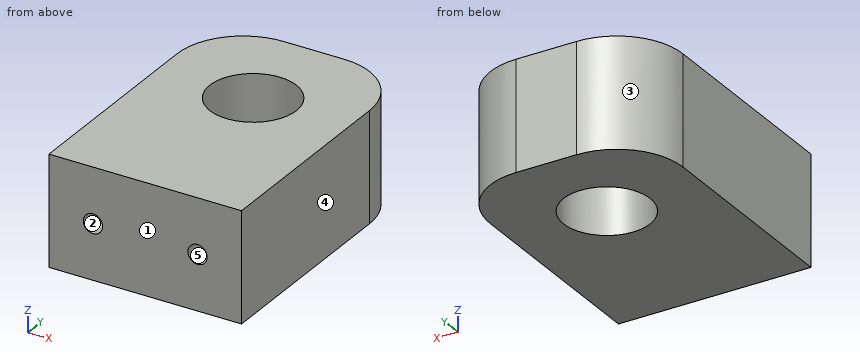
```python
from build123d import *

# Parameters (mm, degrees)
SKETCH1_W           = 35
SKETCH1_H           = 20
BOSS_EXTRUDE1_DEPTH = 50
SKETCH2_R           = 7.875
CUT_EXTRUDE1_DEPTH  = 21
SKETCH3_R           = 1.75
CUT_EXTRUDE2_DEPTH  = 10
FILLET1_R           = 12


with BuildPart() as part:
    # Sketch1 → Boss-Extrude1 (new body)
    with BuildSketch(Plane(origin=(0, 0, 0), x_dir=(1, 0, 0), z_dir=(0, 1, 0))):
        with Locations((1.164675851, -0.855170824)):
            Rectangle(SKETCH1_W, SKETCH1_H)
    extrude(amount=BOSS_EXTRUDE1_DEPTH)

    # Sketch2 → Cut-Extrude1 (cut, through all)
    with BuildSketch(Plane.XY.offset(10.855170824)):
        with Locations((1.164675851, 32)):
            Circle(SKETCH2_R)
    extrude(amount=-CUT_EXTRUDE1_DEPTH, mode=Mode.SUBTRACT)

    # Sketch3 → Cut-Extrude2 (cut)
    with BuildSketch(Plane.XZ):
        with Locations((-8.335324149, 0.855170824)):
            Circle(SKETCH3_R)
        with Locations((10.664675851, 0.855170824)):
            Circle(SKETCH3_R)
    extrude(amount=-CUT_EXTRUDE2_DEPTH, mode=Mode.SUBTRACT)

    # Fillet1
    fillet1_edges = [part.edges().sort_by_distance(p)[0] for p in [
        (18.664675851, 50, 0.855170824),
        (-16.335324149, 50, 0.855170824),
    ]]
    fillet(fillet1_edges, radius=FILLET1_R)


solid = part.part
```
Here's how the part is built. I have some questions about the finished solid (model axes, mm). Face numbers are marked on the shaded views. A direction names the side the tool comes from. Round coordinates to 2 decimals unless told otherwise and drop trailing zeros. Order: outer loops, then holes, each group sorted by start corner. A loop starts at its lowest first (then second) coordinate and runs counter-clockwise, first axis right, second up. Notation, with made-up numbers: (4.25, 67.25) -> (11.25, 67.25) arc R11 ccw to (11.25, 82.25) -> close; hole circle Ø7 at (-37, -14.75). An arc over 180 degrees is marked (long way). Use a Markdown table: item, result. Add a question column.
(1) For the marked faces 4 and 5, which set-ups out of +Z, -Z, +X, -X, +Y, -Y let a thin tool reach every point of the face, with its end or its side?
(2) For pin 1 Ø1.5 at (x, z) = (5, 0.5) entering from -Y; pin 2 Ø1 at (x, z) = (-8, 0) entering from -Y; pin 3 Ø3 at (x, z) = (10.66, 0.86) entering from +Y, each with a flat end and sliding along its axis, tell me the tip position at first contact or that it passes through.
(3) Suppose I cut it at C-C, the plane y = 47. Please give me the cut outline in (x, z), and give its area (3 significant figures).
(4) I need wall thicknesses on line 1 along X through (y, z) = (30, -1); line 2 along Y through (x, z) = (7, -1); line 3 along X through (y, z) = (28, -7.25). Which ranges of each line are inside material? Lowest first, please.
(5) If we mould it in two halves opening along X, with no side actions, what happens to the marked faces 1, 2 and 3? For each: released by +X, released by -X, zero draft, split by the parting line, or undercut.
(6) Suppose I cut it at A-A, the plane y = 32. Please give me the cut outline in (x, z).
(7) Suppose I cut it at B-B, the plane z = 4.25. Please give me the cut outline in (x, y) (3 decimals), and give its area (3 significant figures).
Verdict:
| question | item | result |
|---|---|---|
| 1 | face 4 | +Z, -Z, +X, +Y, -Y |
| 1 | face 5 | -Y |
| 2 | pin 1 | y = 0 |
| 2 | pin 2 | y = 10 |
| 2 | pin 3 | y = 49.74 |
| 3 | outline | (-12.27, -9.14) -> (14.6, -9.14) -> (14.6, 10.86) -> (-12.27, 10.86) -> close |
| 3 | area | 537 mm2 |
| 4 | line 1 | -16.34 to -6.45, 8.78 to 18.66 |
| 4 | line 2 | 0 to 26.71, 37.29 to 50 |
| 4 | line 3 | -16.34 to -5.62, 7.95 to 18.66 |
| 5 | face 1 | zero draft |
| 5 | face 2 | undercut |
| 5 | face 3 | released by -X |
| 6 | outline | (-16.34, -9.14) -> (-6.71, -9.14) -> (-6.71, 10.86) -> (-16.34, 10.86) -> close; (9.04, -9.14) -> (18.66, -9.14) -> (18.66, 10.86) -> (9.04, 10.86) -> close |
| 7 | outline | (-16.335, 0) -> (18.665, 0) -> (18.665, 38) arc R12 ccw to (6.665, 50) -> (-4.335, 50) arc R12 ccw to (-16.335, 38) -> close; hole circle Ø15.75 at (1.165, 32) |
| 7 | area | 1,490 mm2 |
